Here's how the part is built. I have some questions about the finished solid (model axes, mm). Give positions to 0.01 mm unless a question says otherwise; leave off trailing zeros. Loops run counter-clockwise (first coordinate to the right, second up) from the corner with the lowest first, then second, coordinate; pieces in that order, holes last. Notation, with made-up numbers: (52, -19) - (86, -19) arc R19 ccw to (86, 10) - close; hole circle Ø11 at (-32.75, 75.25). An arc over 180 degrees is marked (long way). Use a Markdown table: item, result.
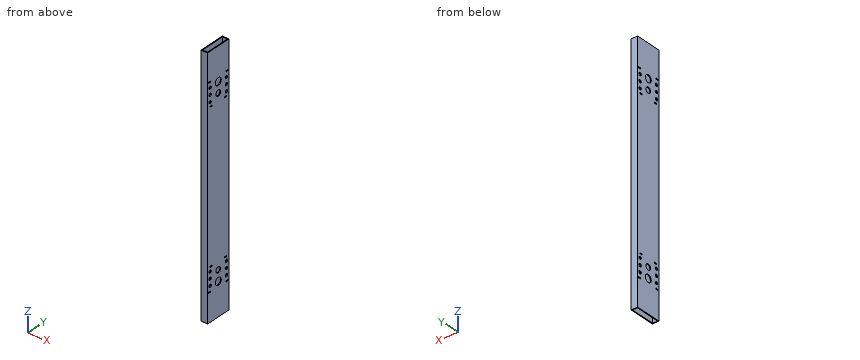
Autodesk Inventor part; units mm, degrees
ref_plane "YZ Plane" through (0, 0, 0) normal (1, 0, 0) x (0, 1, 0)
ref_plane "XZ Plane" through (0, 0, 0) normal (0, 1, 0) x (-1, 0, 0)
ref_plane "XY Plane" through (0, 0, 0) normal (0, 0, 1) x (1, 0, 0)
sketch "Sketch1" plane through (0, 0, 0) normal (0, 1, 0) x (-1, 0, 0)
  line L0 (0, 0) -> (0, -965.2)
  line L1 (0, -965.2) -> (25.4, -965.2)
  line L2 (0, 0) -> (25.4, 0)
  line L3 (25.4, 0) -> (25.4, -965.2)
  dimension "d0" = 965.2
  dimension "d1" = 25.4
  dimension "d2" = 25.4
  dimension "d3" = 965.2
extrude "Extrusion1" add sketch "Sketch1" along normal blind 101.6
sketch "Sketch2" plane through (0, 0, -965.2) normal (0, 0, -1) x (-1, 0, 0)
  line L0 (0, 101.6) -> (25.4, 101.6)
  line L1 (22.225, 98.425) -> (3.175, 98.425)
  line L2 (3.175, 98.425) -> (3.175, 3.175)
  line L3 (3.175, 3.175) -> (22.225, 3.175)
  line L4 (22.225, 3.175) -> (22.225, 98.425)
  point P0 (0, 0)
  dimension "d8" = 19.05
  dimension "d9" = 95.25
  dimension "d10" = 19.05
extrude "Extrusion2" cut sketch "Sketch2" against normal blind 2540
sketch "Sketch3" plane through (-25.4, 0, -965.2) normal (-1, 0, 0) x (0, 0, 1)
  line L0 (89.1033, 114.2993) -> (200.7415, 105.2475)
  arc A0 (206.5783, 98.9183) -> (200.7415, 105.2475) centre (200.2283, 98.9183) ccw
  line L1 (206.5783, 98.9183) -> (206.5783, 2.6802)
  arc A1 (200.7415, -3.649) -> (206.5783, 2.6802) centre (200.2283, 2.6802) ccw
  line L2 (200.7415, -3.649) -> (89.1033, -12.7007)
  line L3 (89.1033, -12.7007) -> (87.4523, -12.7007)
  line L4 (87.4523, 114.2993) -> (87.4523, -12.7007)
  line L5 (87.4523, 114.2993) -> (89.1033, 114.2993)
  circle A2 centre (108.688, 6.2223) radius 2.0447
  circle A3 centre (197.588, 88.3913) radius 2.0447
  circle A4 centre (108.688, 12.0643) radius 2.5527
  circle A5 centre (197.588, 82.5493) radius 2.5527
  circle A6 centre (180.57, 12.0643) radius 5.5562
  circle A7 centre (129.77, 12.0643) radius 5.5562
  circle A8 centre (180.57, 89.5343) radius 5.5562
  circle A9 centre (167.7163, 50.7993) radius 11.1061
  circle A10 centre (155.17, 89.5343) radius 5.5562
  circle A11 centre (129.77, 89.5343) radius 5.5562
  circle A12 centre (155.17, 12.0643) radius 5.5562
  circle A13 centre (127.0001, 50.7993) radius 14.2811
  circle A14 centre (197.588, 19.0493) radius 2.5527
  circle A15 centre (108.688, 89.5343) radius 2.5527
  circle A16 centre (197.588, 13.2073) radius 2.0447
  circle A17 centre (108.688, 95.3763) radius 2.0447
  circle A18 centre (197.588, 13.2073) radius 2.0447
  circle A19 centre (197.588, 19.0493) radius 2.5527
  circle A20 centre (197.588, 82.5493) radius 2.5527
  circle A21 centre (197.588, 88.3913) radius 2.0447
  circle A22 centre (167.7163, 50.7993) radius 11.1061
  circle A23 centre (180.57, 89.5343) radius 5.5563
  circle A24 centre (155.17, 89.5343) radius 5.5562
  circle A25 centre (129.77, 89.5343) radius 5.5562
  circle A26 centre (127.0001, 50.7993) radius 14.2811
  circle A27 centre (129.77, 12.0643) radius 5.5562
  circle A28 centre (155.17, 12.0643) radius 5.5562
  circle A29 centre (180.57, 12.0643) radius 5.5562
  circle A30 centre (108.688, 89.5343) radius 2.5527
  circle A31 centre (108.688, 95.3763) radius 2.0447
  circle A32 centre (108.688, 12.0643) radius 2.5527
  circle A33 centre (108.688, 6.2223) radius 2.0447
  line L6 (0, 101.6) -> (0, 50.8)
  line L7 (965.2, 101.6) -> (965.2, 50.8)
  line L8 (965.2, 3.175) -> (965.2, 98.425)
  line L9 (0, 50.8) -> (127, 50.8)
  line L10 (965.2, 50.8) -> (838.2, 50.8)
  line L11 (965.2, 101.6) -> (0, 101.6)
  line L12 (482.6, 101.6) -> (482.6, 3.175)
  circle A34 centre (767.612, 88.3913) radius 2.0447
  arc A35 (764.4585, 105.2475) -> (758.6217, 98.9183) centre (764.9717, 98.9183) ccw
  circle A36 centre (767.612, 82.5493) radius 2.5527
  circle A37 centre (767.612, 82.5493) radius 2.5527
  line L13 (758.6217, 98.9183) -> (758.6217, 2.6802)
  arc A38 (758.6217, 2.6802) -> (764.4585, -3.649) centre (764.9717, 2.6802) ccw
  circle A39 centre (767.612, 88.3913) radius 2.0447
  circle A40 centre (784.63, 89.5343) radius 5.5562
  circle A41 centre (784.63, 89.5343) radius 5.5563
  circle A42 centre (810.03, 89.5343) radius 5.5562
  circle A43 centre (810.03, 89.5343) radius 5.5562
  line L14 (764.4585, -3.649) -> (876.0967, -12.7007)
  line L15 (877.7477, 114.2993) -> (877.7477, -12.7007)
  circle A44 centre (835.43, 89.5343) radius 5.5562
  circle A45 centre (835.43, 89.5343) radius 5.5562
  line L16 (876.0967, 114.2993) -> (764.4585, 105.2475)
  circle A46 centre (856.512, 95.3763) radius 2.0447
  circle A47 centre (856.512, 95.3763) radius 2.0447
  circle A48 centre (856.512, 89.5343) radius 2.5527
  circle A49 centre (856.512, 89.5343) radius 2.5527
  line L17 (877.7477, 114.2993) -> (876.0967, 114.2993)
  line L18 (876.0967, -12.7007) -> (877.7477, -12.7007)
  circle A50 centre (856.512, 6.2223) radius 2.0447
  circle A51 centre (856.512, 12.0643) radius 2.5527
  circle A52 centre (856.512, 6.2223) radius 2.0447
  circle A53 centre (856.512, 12.0643) radius 2.5527
  circle A54 centre (835.43, 12.0643) radius 5.5562
  circle A55 centre (835.43, 12.0643) radius 5.5562
  circle A56 centre (838.1999, 50.7993) radius 14.2811
  circle A57 centre (838.1999, 50.7993) radius 14.2811
  circle A58 centre (810.03, 12.0643) radius 5.5562
  circle A59 centre (810.03, 12.0643) radius 5.5562
  circle A60 centre (784.63, 12.0643) radius 5.5562
  circle A61 centre (784.63, 12.0643) radius 5.5562
  circle A62 centre (767.612, 13.2073) radius 2.0447
  circle A63 centre (767.612, 13.2073) radius 2.0447
  circle A64 centre (767.612, 19.0493) radius 2.5527
  circle A65 centre (767.612, 19.0493) radius 2.5527
  circle A66 centre (797.4837, 50.7993) radius 11.1061
  circle A67 centre (797.4837, 50.7993) radius 11.1061
  point P0 (965.2, 0)
  point P1 (758.7399, 264.0927)
  point P2 (0, 76.2)
  dimension "d13" = 50.8
  dimension "d15" = 50.8
  dimension "d216" = 127
  dimension "d217" = 127
extrude "Extrusion7" cut sketch "Sketch3" against normal blind 2540 contours A13
extrude "Extrusion8" cut sketch "Sketch3" against normal blind 2540 contours A2 | A3 | A4 | A5 | A6 | A7 | A8 | A9 | A10 | A11 | A12 | A14 | A15 | A16 | A17
extrude "Extrusion11" cut sketch "Sketch3" against normal through all contours A56 | A13 | A2 | A3 | A4 | A5 | A6 | A7 | A8 | A9 | A10 | A11 | A12 | A14 | A15 | A16 | A17 | A34 | A36 | A40 | A42 | A44 | A46 | A48 | A50 | A51 | A54 | A58 | A60 | A62 | A64 | A66
properties part number "boxbeam 4x1 with sideways holes"
(1) Will this pin go through, and if not, where does the flat tip stop? pin 1 (3.5 mm diameter, centred on y = 88.39, z = -197.59, fed in from +X).
A:
| item | result |
|---|---|
| pin 1 | through |
(2) If I drill on line 1 (Z direction, x = -24, y = 50.5); line 2 (X direction, y = 92, z = -891) (3 decimals); line 3 (Y direction, x = -23.8, z = -180.57), over which ranges is the centre line in solid material (lowest first)?
A:
| item | result |
|---|---|
| line 1 | -965.2 to -852.48, -823.92 to -808.59, -786.38 to -178.82, -156.61 to -141.28, -112.72 to 0 |
| line 2 | -25.4 to -22.225, -3.175 to 0 |
| line 3 | 0 to 6.51, 17.62 to 83.98, 95.09 to 101.6 |
(3) Suppose I cut it at B-B on x = -8.25. Write out the boundary of the cut face in (y, z) (3 decimals), plus the area to 3 significant figures.
A:
| item | result |
|---|---|
| outline | (0, -965.2) - (3.175, -965.2) - (3.175, 0) - (0, 0) - close; (98.425, -965.2) - (101.6, -965.2) - (101.6, 0) - (98.425, 0) - close |
| area | 6,130 mm2 |
(4) Suppose I cut it at A-A on z = -264.5. Write out the boundary of the cut face in (x, y) (3 decimals).
A:
| item | result |
|---|---|
| outline | (-25.4, 0) - (0, 0) - (0, 101.6) - (-25.4, 101.6) - close; hole (-22.225, 3.175) - (-3.175, 3.175) - (-3.175, 98.425) - (-22.225, 98.425) - close |
